from build123d import *

# Parameters (mm, degrees)
SKETCH_1_W               = 12.5
SKETCH_1_H               = 19.2
EXTRUDE_1_DEPTH          = 13
SKETCH_2_W               = 5
SKETCH_2_H               = 1
EXTRUDE_2_DEPTH          = 9
CHAMFER_1_SIZE           = 1
CUT_EXTRUDE_1_DEPTH      = 18.608875603
CUT_EXTRUDE_1_DEPTH_BACK = 18.608875603
SKETCH_4_W               = 15.2
SKETCH_4_H               = 21.5
EXTRUDE_3_DEPTH          = 2
EXTRUDE_4_DEPTH          = 5


with BuildPart() as part:
    # Эскиз1 → Бобышка-Вытянуть1 (new body)
    with BuildSketch(Plane(origin=(0, 0, 0), x_dir=(1, 0, 0), z_dir=(0, 1, 0))):
        Rectangle(SKETCH_1_W, SKETCH_1_H)
    extrude(amount=EXTRUDE_1_DEPTH)

    # Эскиз2 → Бобышка-Вытянуть2 (add)
    with BuildSketch(Plane.XZ):
        Rectangle(SKETCH_2_W, SKETCH_2_H)
        with Locations((0, 5)):
            Rectangle(SKETCH_2_W, SKETCH_2_H)
    extrude(amount=EXTRUDE_2_DEPTH)

    # Фаска1
    chamfer_1_edges = [part.edges().sort_by_distance(p)[0] for p in [
        (2.5, -9, 5),
        (-2.5, -9, 5),
        (2.5, -9, 0),
        (-2.5, -9, 0),
    ]]
    chamfer(chamfer_1_edges, length=CHAMFER_1_SIZE)

    # Эскиз3 → Вырез-Вытянуть1 (cut, two sides: drawn at the far end of the back side and taken through both)
    with BuildSketch(Plane(origin=(0, 0, -0.5), x_dir=(-1, 0, 0), z_dir=(0, 0, -1)).offset(-CUT_EXTRUDE_1_DEPTH_BACK)):
        with BuildLine():
            Line((0.942809042, -4.833333333), (0.471404521, -6.166666667))
            ThreePointArc((0.471404521, -6.166666667), (0, -6.5), (-0.471404521, -6.166666667))
            Line((-0.471404521, -6.166666667), (-0.942809042, -4.833333333))
            ThreePointArc((-0.942809042, -4.833333333), (0, -3.5), (0.942809042, -4.833333333))
        make_face()
    extrude(amount=CUT_EXTRUDE_1_DEPTH + CUT_EXTRUDE_1_DEPTH_BACK, mode=Mode.SUBTRACT)

    # Эскиз4 → Бобышка-Вытянуть3 (add)
    with BuildSketch(Plane(origin=(0, 13, 0), x_dir=(1, 0, 0), z_dir=(0, 1, 0))):
        Rectangle(SKETCH_4_W, SKETCH_4_H)
    extrude(amount=EXTRUDE_3_DEPTH)

    # Эскиз5 → Бобышка-Вытянуть4 (add, symmetric)
    with BuildSketch(Plane(origin=(0, 0, 0), x_dir=(0, 0, -1), z_dir=(1, 0, 0))):
        with BuildLine():
            Line((-7, 15), (7, 15))
            Line((7, 15), (5.451254755, 18.321294895))
            ThreePointArc((5.451254755, 18.321294895), (-0.556694467, 15.844590382), (-7, 15))
        make_face()
    extrude(amount=EXTRUDE_4_DEPTH, both=True)


solid = part.part
Can you work these out from the model? Positions are in its coordinate system, mm. A direction names the side the tool comes from. Coordinates: 2 decimals unless noted, no trailing zeros. Loops run counter-clockwise (first coordinate to the right, second up) from the corner with the lowest first, then second, coordinate; pieces in that order, holes last. Notation, with made-up numbers: (84, 61.25) - (105, 61.25) arc R21 ccw to (105, 96.25) - close; hole circle Ø2 at (-29, -37.5). An arc over 180 degrees is marked (long way). Put each result on its own line as item: value. Start each with the question number.
Item 1: Suppose I cut it at A-A (x = 0). Please give me the cut outline in (y, z), and give its area (3 significant figures).
Item 2: Suppose I cut it at C-C (x = 2). Please give me the cut outline in (y, z), and give its area (3 significant figures).
Item 3: If we mould it in two halves opening along Y, with no side actions, what happens to faces 6 (the face through (0, -3, 4.5)), 7 (the face through (0, 16, 0)), 8 (the face through (0, -3.5, 5)), 9 (the face through (0, 0, -2))? For each: +Y half, -Y half, draft (parallel to the pull), parting line (faces both ways), or undercut.
Item 4: Suppose I cut it at B-B (y = -2.5). Please give me the cut outline in (x, z), and give its area (3 significant figures).
Item 5: Suppose I cut it at D-D (z = 8.25). Please give me the cut outline in (x, y).
Item 6: Which directions (+Z, -Z, +X, -X, +Y, -Y) give clear straight access to the entire face, cutting with the end or side of a thin tool? Please do faces 1 (the face through (0, 6, -9.6)), 2 (the face through (0.704, -5.509, 0.007)), 3 (the face through (7.6, 14, 0)), 4 (the face through (0, 6, 9.6)), 5 (the face through (2.5, -4, 5)).
Item 7: If I drill on line 1 along X through (y, z) = (-4.5, 0.05); line 2 along X through (y, z) = (16.25, -6.25); line 3 along Y through (x, z) = (-5.25, -2.5), over which ranges is the centre line in solid material (lowest first)?
Item 8: For pin 1 (0.5 mm diameter, centred on y = -3.5, z = 0, fed in from -X); pin 2 (1 mm diameter, centred on y = 16, z = 0.5, fed in from +X); pin 3 (3 mm diameter, centred on x = 5, z = -5.5, fed in from -Y), each with a flat end and sliding along its axis, tell me the tip position at first contact or that it passes through.
Here are the results:
1. outline: (-9, -0.5) - (-6.5, -0.5) - (-6.5, 0.5) - (-9, 0.5) - close; (-9, 4.5) - (-6.5, 4.5) - (-6.5, 5.5) - (-9, 5.5) - close; (-3.5, -0.5) - (0, -0.5) - (0, -9.6) - (13, -9.6) - (13, -10.75) - (15, -10.75) - (15, -7) - (18.32, -5.45) arc R25 cw to (15, 7) - (15, 10.75) - (13, 10.75) - (13, 9.6) - (0, 9.6) - (0, 5.5) - (-3.5, 5.5) - (-3.5, 4.5) - (0, 4.5) - (0, 0.5) - (-3.5, 0.5) - close
1. area: 321 mm²
2. outline: (-8.5, -0.5) - (0, -0.5) - (0, -9.6) - (13, -9.6) - (13, -10.75) - (15, -10.75) - (15, -7) - (18.32, -5.45) arc R25 cw to (15, 7) - (15, 10.75) - (13, 10.75) - (13, 9.6) - (0, 9.6) - (0, 5.5) - (-8.5, 5.5) - (-8.5, 4.5) - (0, 4.5) - (0, 0.5) - (-8.5, 0.5) - close
2. area: 326 mm²
3. face 6: draft
3. face 7: +Y half
3. face 8: undercut
3. face 9: -Y half
4. outline: (-2.5, -0.5) - (2.5, -0.5) - (2.5, 0.5) - (-2.5, 0.5) - close; (-2.5, 4.5) - (2.5, 4.5) - (2.5, 5.5) - (-2.5, 5.5) - close
4. area: 10.0 mm²
5. outline: (-7.6, 13) - (-6.25, 13) - (-6.25, 0) - (6.25, 0) - (6.25, 13) - (7.6, 13) - (7.6, 15) - (-7.6, 15) - close
6. face 1: -Z, +X, -X, -Y
6. face 2: +Z, -Z
6. face 3: +Z, -Z, +X, +Y, -Y
6. face 4: +Z, +X, -X, -Y
6. face 5: +Z, -Z, +X, -Y
7. line 1: -2.5 to -1, 1 to 2.5
7. line 2: -5 to 5
7. line 3: 0 to 15
8. pin 1: x = -2.5
8. pin 2: x = 5
8. pin 3: y = 0
